from build123d import *

# Parameters (mm, degrees)
F0_W        = 40
F0_H        = 40
F0_W_2      = 36
F0_H_2      = 36
F1_DEPTH    = 1430
F2_T1_DEPTH = 245.7346390373


# Not quite as in the source:
# - a fillet or chamfer that OpenCascade refuses, or shapes differently, is made with other operations: its cross-section is extruded or revolved along the edge and cut away or added


with BuildPart() as f1:
    # F0 (on Top) → F1 (new body)
    with BuildSketch(Plane.XY):
        with Locations((20, 20)):
            Rectangle(F0_W, F0_H)
        with Locations((20, 20)):
            Rectangle(F0_W_2, F0_H_2, mode=Mode.SUBTRACT)
    extrude(amount=F1_DEPTH)

    # F2: chamfer of 40 on 2 edges, made by hand

    # F2_s2 → F2_t1 (cut)
    with BuildSketch(Plane.XZ.offset(-142.8673195186)):
        Polygon((0, 40), (40, 0), (0, 0), align=None)
        Polygon((0, 1390), (40, 1430), (0, 1430), align=None)
    extrude(amount=F2_T1_DEPTH, mode=Mode.SUBTRACT)


solid = f1.part
Check sheet for the modelled part. Datum: model origin and axes. Units: mm. A direction names the side the tool comes from. Give positions to 0.01 mm unless a question says otherwise; leave off trailing zeros. Order: outer loops, then holes, each group sorted by start corner. A loop starts at its lowest first (then second) coordinate and runs counter-clockwise, first axis right, second up. Notation, with made-up numbers: M 45,-33.5 L 95,-33.5 A24 cw 95,-6.5 Z; hole C 52,53 d11. An arc over 180 degrees is marked long. Answer as CSV lines item,"result". Start each with the question number.
Item 1: Thickness scan on line 1 (Y direction, x = 7.5, z = 200). Record the ranges inside material, lowest first. Write a range as [from, to].
Item 2: Mould release check, pull along Y, two halves, no side actions. Record for faces 1 (the face through (20, 0, 705)), 2 (the face through (18, 1, 22)), 3 (the face through (2, 20, 706)), 4 (the face through (38, 20, 705)): +Y half, -Y half, draft (parallel to the pull), parting line (faces both ways), or undercut.
Item 3: Cross-section at C-C on z = 1299.5. Enter the section's corners in (x, y), plus the area to 3 significant figures.
Item 4: Cross-section at B-B on y = 31.5. Enter the section's corners in (x, z).
Item 5: Tool access check on faces 5 (the face through (40, 20, 705)), 6 (the face through (20, 38, 705)). Record the directions out of +Z, -Z, +X, -X, +Y, -Y that give a thin tool (end or side, any length) a straight path to the whole face; none if there is none.
Item 6: Cross-section at A-A on x = 19. Enter the section's corners in (y, z), plus the area to 3 significant figures.
Established:
1,line 1,"y = [0, 2], [38, 40]"
2,face 1,"-Y half"
2,face 2,"draft"
2,face 3,"undercut"
2,face 4,"undercut"
3,outline,"M 0,0 L 40,0 L 40,40 L 0,40 Z; hole M 2,2 L 38,2 L 38,38 L 2,38 Z"
3,area,"304 mm^2"
4,outline,"M 0,40 L 2,38 L 2,1392 L 0,1390 Z; M 38,2 L 40,0 L 40,1430 L 38,1428 Z"
5,face 5,"+Z, -Z, +X, +Y, -Y"
5,face 6,"+Z, -Z"
6,outline,"M 0,21 L 2,21 L 2,1409 L 0,1409 Z; M 38,21 L 40,21 L 40,1409 L 38,1409 Z"
6,area,"5,550 mm^2"
